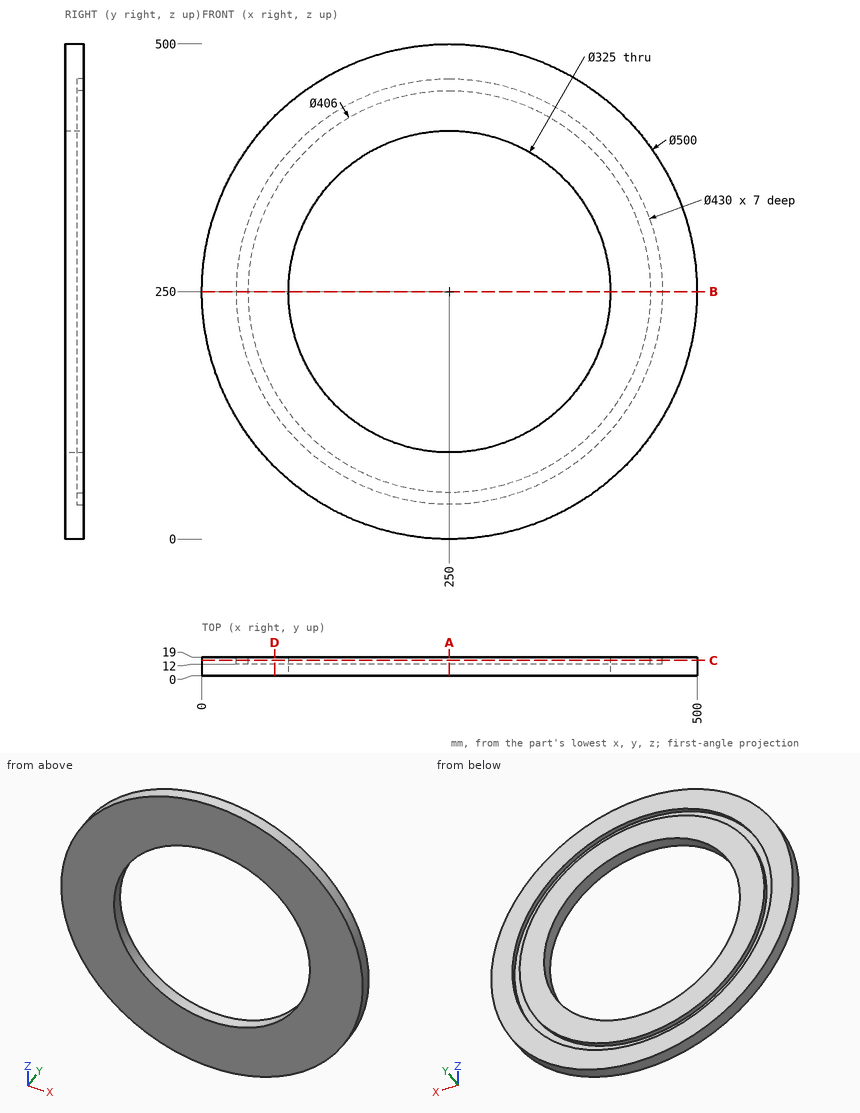
Here's the drawing with two shaded views (mm, measured from the low corner). I have some questions. Round coordinates to 2 decimals unless told otherwise and drop trailing zeros. Loops run counter-clockwise (first coordinate to the right, second up) from the corner with the lowest first, then second, coordinate; pieces in that order, holes last.
1. Suppose I cut it at D-D, the plane x = 73.5. Please give me the cut outline in (y, z).
Answers:
outline: (0, 72.95) - (19, 72.95) - (19, 127.23) - (12, 127.23) - (12, 149.72) - (19, 149.72) - (19, 350.28) - (12, 350.28) - (12, 372.77) - (19, 372.77) - (19, 427.05) - (0, 427.05) - close
2. Suppose I cut it at A-A, the plane x = 250. Please give me the cut outline in (y, z), and give its area (3 significant figures).
Answers:
outline: (0, 0) - (19, 0) - (19, 35) - (12, 35) - (12, 47) - (19, 47) - (19, 87.5) - (0, 87.5) - close; (0, 412.5) - (19, 412.5) - (19, 453) - (12, 453) - (12, 465) - (19, 465) - (19, 500) - (0, 500) - close
area: 3,160 mm2
3. If I drill on probe 1 along X at (y, z) = (14, 250); probe 2 along X at (y, z) = (13.75, 424); probe 3 along X at (y, z) = (6.75, 250), over which ranges is the centre line in solid material (lowest first)?
Answers:
probe 1: x = 0 to 35, 47 to 87.5, 412.5 to 453, 465 to 500
probe 2: x = 70.49 to 123.71, 145.44 to 354.56, 376.29 to 429.51
probe 3: x = 0 to 87.5, 412.5 to 500
4. Will these pins go through, and if not, where does the flat tip stop? pin 1 (10 mm diameter, centred on x = 405, y = 9, fed in from +Z); pin 2 (3 mm diameter, centred on x = 184, y = 11.5, fed in from -Z); pin 3 (4 mm diameter, centred on y = 14.5, z = 97, fed in from +X).
Answers:
pin 1: stops at z = 450
pin 2: stops at z = 8.46
pin 3: stops at x = 449.25
5. Suppose I cut it at B-B, the plane z = 250. Please give me the cut outline in (x, y), and give its area (3 significant figures).
Answers:
outline: (0, 0) - (87.5, 0) - (87.5, 19) - (47, 19) - (47, 12) - (35, 12) - (35, 19) - (0, 19) - close; (412.5, 0) - (500, 0) - (500, 19) - (465, 19) - (465, 12) - (453, 12) - (453, 19) - (412.5, 19) - close
area: 3,160 mm2
6. Suppose I cut it at C-C, the plane y = 15.75. Please give me the cut outline in (x, z).
Answers:
outline: circle Ø500 at (250, 250); circle Ø406 at (250, 250); hole circle Ø430 at (250, 250); hole circle Ø325 at (250, 250)
